Could you check a few things on this model? Use its own coordinates, in mm. Face numbers are marked on the shaded views. Coordinates: 2 decimals unless noted, no trailing zeros. Use a Markdown table: item, result. Add a question column.
1) Thinking about a two-plate mould opening in X: for the marked faces 1, 2 and 3, which applies, +X half, -X half, draft (parallel to the pull), parting line (faces both ways), or undercut?
2) Will these pins go through, and if not, where does the flat tip stop? pin 1 Ø12 at (x, y) = (62, 8.5) entering from +Z; pin 2 Ø4 at (x, z) = (73.34, -7.94) entering from -Y.
3) If we section it at A-A (y = 22.75): Give the number of separate pieces and of enclosed holes in the cut face, plus the area to 3 significant figures.
4) If I drill on L1, parallel to Z at x = 136.5, y = 8.5 (3 decimals); L2, parallel to X at y = 20.75, z = -7.5; L3, parallel to X at y = 19.75, z = -12.75, over which ranges is the centre line in solid material (lowest first)? Write a range as [from, to].
Autodesk Inventor part; units mm, degrees
ref_plane "YZ Plane" through (0, 0, 0) normal (1, 0, 0) x (0, 1, 0)
ref_plane "XZ Plane" through (0, 0, 0) normal (0, 1, 0) x (-1, 0, 0)
ref_plane "XY Plane" through (0, 0, 0) normal (0, 0, 1) x (1, 0, 0)
sketch "Sketch1" plane through (0, 0, 0) normal (1, 0, 0) x (0, 1, 0)
  line L0 (0, 0) -> (25.4, 0)
  line L1 (25.4, 0) -> (25.4, -15.875)
  line L2 (25.4, -15.875) -> (0, -15.875)
  line L3 (0, -15.875) -> (0, 0)
  dimension "d0" = 25.4
  dimension "d1" = 15.875
extrude "Extrusion1" add sketch "Sketch1" along normal blind 144.78
chamfer "Chamfer1" distance 0.762 angle 45 11 edges at (144.78, 12.7, 0) (144.78, 12.7, -15.875) (144.78, 0, -7.9375) (72.39, 0, 0) (72.39, 25.4, 0) (72.39, 25.4, -15.875) (0, 12.7, 0) (0, 25.4, -7.9375) (0, 12.7, -15.875) (0, 0, -7.9375) (72.39, 0, -15.875)
sketch "Sketch2" plane through (0.762, 25.4, -15.113) normal (0, 1, 0) x (1, 0, 0)
  line L0 (0, -15.113) -> (143.256, -15.113)
  line L1 (0, -15.113) -> (7.9375, -15.113)
  line L2 (7.9375, -15.113) -> (7.9375, -7.1755)
  point P0 (-0.762, -15.113)
  dimension "d7" = 7.9375
  dimension "d8" = 7.9375
hole "Hole1" at (8.6995, 25.4, -7.9375) direction (0, -1, 0) diameter 7.9375 end through all countersink diameter 9.525 countersink angle 82
sketch "Sketch3" plane through (0.762, 25.4, -15.113) normal (0, 1, 0) x (1, 0, 0)
  line L0 (144.018, 0) -> (144.018, -14.351)
  line L1 (144.018, -7.1755) -> (72.5805, -7.1755)
  point P0 (-0.762, -15.113)
  dimension "d16" = 71.4375
hole "Hole2" at (73.3425, 25.4, -7.9375) direction (0, -1, 0) diameter 6.35 end through all countersink diameter 7.9375 countersink angle 82
sketch "Sketch4" plane through (0.762, 25.4, -15.113) normal (0, 1, 0) x (1, 0, 0)
  line L0 (144.018, 0) -> (144.018, -14.351)
  line L1 (144.018, -7.1755) -> (90.043, -7.1755)
  point P0 (-0.762, -15.113)
  dimension "d24" = 53.975
hole "Hole3" at (90.805, 25.4, -7.9375) direction (0, -1, 0) diameter 11.1125 end through all countersink diameter 12.7 countersink angle 82
sketch "Sketch5" plane through (0.762, 25.4, -15.113) normal (0, 1, 0) x (1, 0, 0)
  line L0 (144.018, 0) -> (144.018, -14.351)
  line L1 (144.018, -7.1755) -> (136.0805, -7.1755)
  point P0 (-0.762, -15.113)
  dimension "d32" = 7.9375
hole "Hole4" at (136.8425, 25.4, -7.9375) direction (0, -1, 0) diameter 7.9375 end through all countersink diameter 9.525 countersink angle 82
sketch "Sketch6" plane through (0.762, 0.762, 0) normal (0, 0, 1) x (1, 0, 0)
  line L0 (111.9534, -0.762) -> (111.9534, 4.8006) construction
  line L1 (117.1134, 4.8006) -> (90.1259, 4.8006) construction
  point P0 (-0.762, -0.762)
  dimension "d40" = 5.5626
  dimension "d41" = 26.9875
hole "Hole5" at (90.8879, 5.5626, 0) direction (0, 0, -1) diameter 4.7625 end through all countersink diameter 6.35 countersink angle 82
sketch "Sketch7" plane through (0.762, 0.762, 0) normal (0, 0, 1) x (1, 0, 0)
  line L0 (114.57, -0.762) -> (114.57, 16.7005)
  line L1 (116.5466, 16.7005) -> (75.2716, 16.7005)
  point P0 (-0.762, -0.762)
  dimension "d49" = 17.4625
  dimension "d50" = 41.275
hole "Hole6" at (76.0336, 17.4625, 0) direction (0, 0, -1) diameter 6.35 end through all countersink diameter 7.9375 countersink angle 82
chamfer "Chamfer2" distance 0.762 angle 45 1 edges at (144.78, 25.4, -7.9375)
properties part number "holes1"
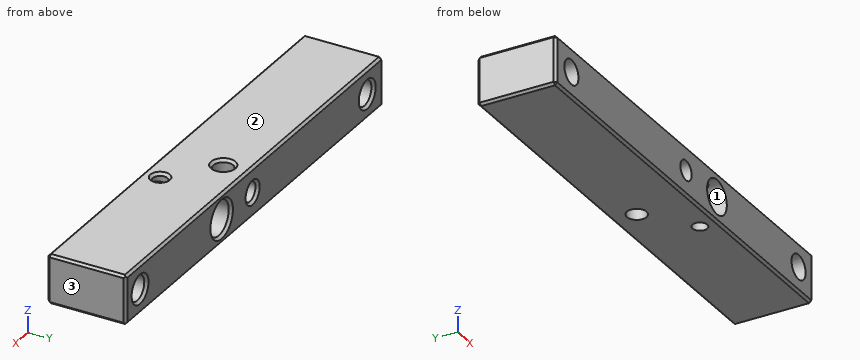
Answer sheet:
| question | item | result |
|---|---|---|
| 1 | face 1 | undercut |
| 1 | face 2 | draft |
| 1 | face 3 | +X half |
| 2 | pin 1 | z = 0 |
| 2 | pin 2 | through |
| 3 | separate pieces | 1 |
| 3 | enclosed holes | 4 |
| 3 | area | 2,070 mm2 |
| 4 | L1 | [-15.875, -11.891], [-3.984, 0] |
| 4 | L2 | [0, 4.75], [12.64, 70.2], [76.49, 85.27], [96.34, 132.9], [140.79, 144.78] |
| 4 | L3 | [0, 73.83], [78.24, 88.03], [93.58, 144.78] |
